Verification items for the finished model (mm, model axes). Face numbers are marked on the shaded views. A direction names the side the tool comes from. Coordinates: 2 decimals unless noted, no trailing zeros. Order: outer loops, then holes, each group sorted by start corner. A loop starts at its lowest first (then second) coordinate and runs counter-clockwise, first axis right, second up. Notation, with made-up numbers: M 35,65 L 69,65 A25 ccw 69,77 Z; hole C 70.25,10.25 d4. An arc over 180 degrees is marked long. Answer as a JSON object with one key per item and string values. Group by question number.
(1) Gauge pin test, flat ends, axial feed: pin 1 Ø5 at (x, y) = (-30.5, -10.5) entering from +Z; pin 2 Ø4 at (x, y) = (12.5, -20) entering from -Z; pin 3 Ø12 at (x, y) = (-7, -11.5) entering from +Z. Record the tip position at first contact, or that the pin passes through.
(2) Cross-section at A-A (x = 17.5). Enter the section's corners in (y, z), plus the area to 3 significant figures.
(3) Cross-section at C-C (y = -9.5). Enter the section's corners in (x, z) (3 decimals), plus the area to 3 significant figures.
(4) Material ranges on line 1 (Z direction, x = 10, y = -15.75); line 2 (Z direction, x = 29.5, y = -16); line 3 (X direction, y = -8, z = 39), recorded low to high.
(5) Access from +Z, -Z, +X, -X, +Y, -Y to the whole of each face (thin tool, end or side, straight path). Record for the marked faces 4 and 5.
(6) Cross-section at B-B (z = 16.5). Enter the section's corners in (x, y).
(7) Mould release check, pull along Z, two halves, no side actions. Record for the marked faces 1, 2 and 3: released by +Z, released by -Z, zero draft, split by the parting line, or undercut.
(8) Cross-section at D-D (z = -39). Enter the section's corners in (x, y), plus the area to 3 significant figures.
from build123d import *

# Parameters (mm, degrees)
F0_R     = 59.886872
F0_R_2   = 16.913856
F0_R_3   = 18.643696
F1_DEPTH = 25.4


with BuildPart() as f1:
    # F0 (on Front) → F1 (new body)
    with BuildSketch(Plane.XZ):
        Circle(F0_R)
        with BuildLine():
            ThreePointArc((32.801818, -17.587269), (-1.953813, -43.724895), (-37.324231, -18.425429))
            ThreePointArc((-37.324231, -18.425429), (-2.125486, -29.361637), (32.801818, -17.587269))
        make_face(mode=Mode.SUBTRACT)
        Polygon((4.024993, -8.088123), (-13.296979, -9.20567), (-3.239061, 8.954463), align=None, mode=Mode.SUBTRACT)
        with Locations((-23.913672, 29.070303)):
            Circle(F0_R_2, mode=Mode.SUBTRACT)
        with Locations((17.156165, 29.349688)):
            Circle(F0_R_3, mode=Mode.SUBTRACT)
    extrude(amount=F1_DEPTH)


solid = f1.part
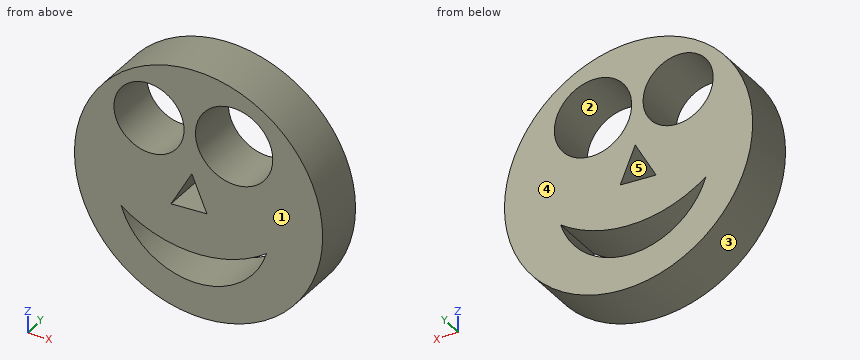
Taken from the geometry:
{
 "1": {"pin 1": "stops at z = 52.94", "pin 2": "stops at z = -58.96", "pin 3": "stops at z = 59.88"},
 "2": {"outline": "M -25.4,-57.27 L 0,-57.27 L 0,-37.88 L -25.4,-37.88 Z; M -25.4,-25.8 L 0,-25.8 L 0,10.71 L -25.4,10.71 Z; M -25.4,47.99 L 0,47.99 L 0,57.27 L -25.4,57.27 Z", "area": "1,660 mm²"},
 "3": {"outline": "C 0,0 d119.774; hole C -23.914,29.07 d33.828; hole M -37.324,-18.425 A36.763 ccw 32.802,-17.587 A59.816 cw Z; hole M -13.297,-9.206 L 4.025,-8.088 L -3.239,8.954 Z; hole C 17.156,29.35 d37.287", "area": "8,340 mm²"},
 "4": {"line 1": "z = -59.05 to -41.58, -27.97 to 12.13, 46.57 to 59.05", "line 2": "z = -52.12 to -25.25, -19.87 to 15.38, 43.32 to 52.12", "line 3": "x = -45.45 to -37.61, -10.22 to 1.2, 33.11 to 45.45"},
 "5": {"face 4": "+Z, -Z, +X, -X, +Y", "face 5": "+Y, -Y"},
 "6": {"outline": "M -57.57,-25.4 L -35.23,-25.4 L -35.23,0 L -57.57,0 Z; M -12.6,-25.4 L 3.65,-25.4 L 3.65,0 L -12.6,0 Z; M 30.66,-25.4 L 57.57,-25.4 L 57.57,0 L 30.66,0 Z"},
 "7": {"face 1": "zero draft", "face 2": "undercut", "face 3": "split by the parting line"},
 "8": {"outline": "M -45.45,-25.4 L -20.43,-25.4 L -20.43,0 L -45.45,0 Z; M 15.64,-25.4 L 45.45,-25.4 L 45.45,0 L 15.64,0 Z", "area": "1,390 mm²"}
}
